Could you check a few things on this drawing? It's one solid part, dimensions in mm from its lowest x, y, z. Give positions to 0.01 mm unless a question says otherwise; leave off trailing zeros. Order: outer loops, then holes, each group sorted by start corner. A loop starts at its lowest first (then second) coordinate and runs counter-clockwise, first axis right, second up. Notation, with made-up numbers: M -34,84 L -3,84 A21 ccw -3,115 Z; hole C 6.25,76 d11. An arc over 180 degrees is marked long. Return JSON: item names as keys, results as strings. Group by question number.
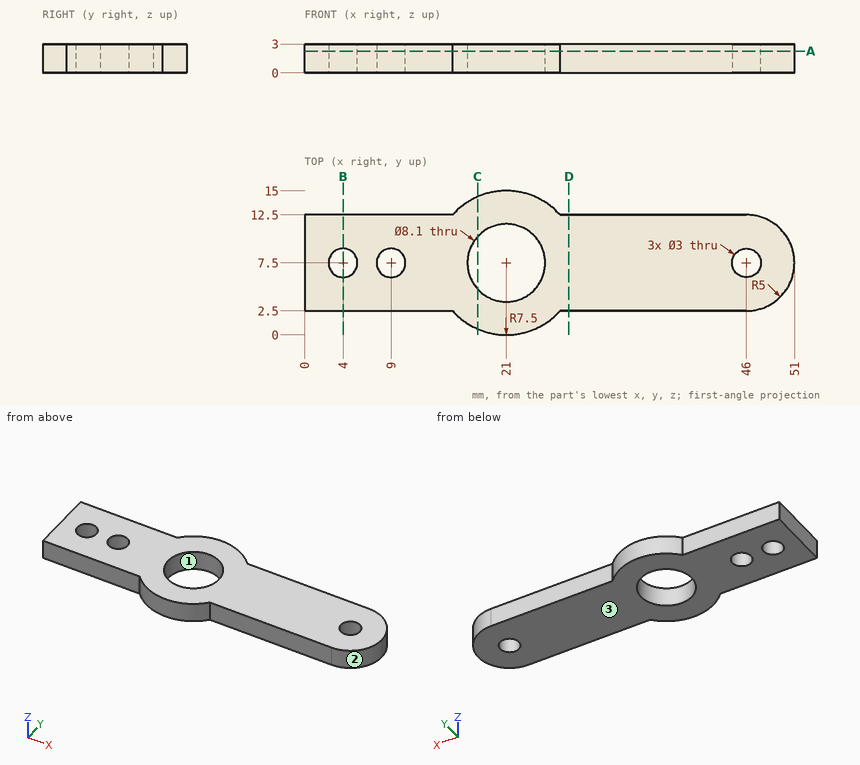
1. If we mould it in two halves opening along Y, with no side actions, what happens to the marked faces 1, 2 and 3? For each: pulls with the +Y half, pulls with the -Y half, needs draft (parallel to the pull), parting line crosses it, or undercut.
2. Imagine slicing it at A-A, the plane z = 2.25. Count the separate pieces of the cut face and the enclosed holes in it, plus the area to 3 significant figures.
3. Imagine slicing it at B-B, the plane x = 4. Please give me the cut outline in (y, z), plus the area to 3 significant figures.
4. Imagine slicing it at C-C, the plane x = 18. Please give me the cut outline in (y, z).
5. I need wall thicknesses on L1, parallel to Y at x = 4, z = 0.75; L2, parallel to Y at x = 39, z = 1.05; L3, parallel to X at y = 10.75, z = 1.35. Which ranges of each line are inside material? Lowest first, please. Write a range as from..to.
6. For pin 1 (5 mm diameter, centred on x = 9, y = 7.5, fed in from -Z); pin 2 (1 mm diameter, centred on y = 9, z = 1, fed in from +X); pin 3 (0.9 mm diameter, centred on x = 41, z = 2, fed in from +Y); pin 4 (0.9 mm diameter, centred on x = 7, z = 2, fed in from -Y), each with a flat end and sliding along its axis, tell me the tip position at first contact or that it passes through.
7. Imagine slicing it at D-D, the plane x = 27.5. Please give me the cut outline in (y, z), plus the area to 3 significant figures.
Values:
{
 "1": {"face 1": "undercut", "face 2": "pulls with the -Y half", "face 3": "needs draft"},
 "2": {"separate pieces": "1", "enclosed holes": "4", "area": "465 mm²"},
 "3": {"outline": "M 2.5,0 L 6,0 L 6,3 L 2.5,3 Z; M 9,0 L 12.5,0 L 12.5,3 L 9,3 Z", "area": "21.0 mm²"},
 "4": {"outline": "M 0.63,0 L 4.78,0 L 4.78,3 L 0.63,3 Z; M 10.22,0 L 14.37,0 L 14.37,3 L 10.22,3 Z"},
 "5": {"L1": "y = 2.5..6, 9..12.5", "L2": "y = 2.5..12.5", "L3": "x = 0..18.58, 23.42..49.8"},
 "6": {"pin 1": "stops at z = 0", "pin 2": "stops at x = 50.9", "pin 3": "stops at y = 12.5", "pin 4": "stops at y = 2.5"},
 "7": {"outline": "M 2.5,0 L 12.5,0 L 12.5,3 L 2.5,3 Z", "area": "30.0 mm²"}
}
